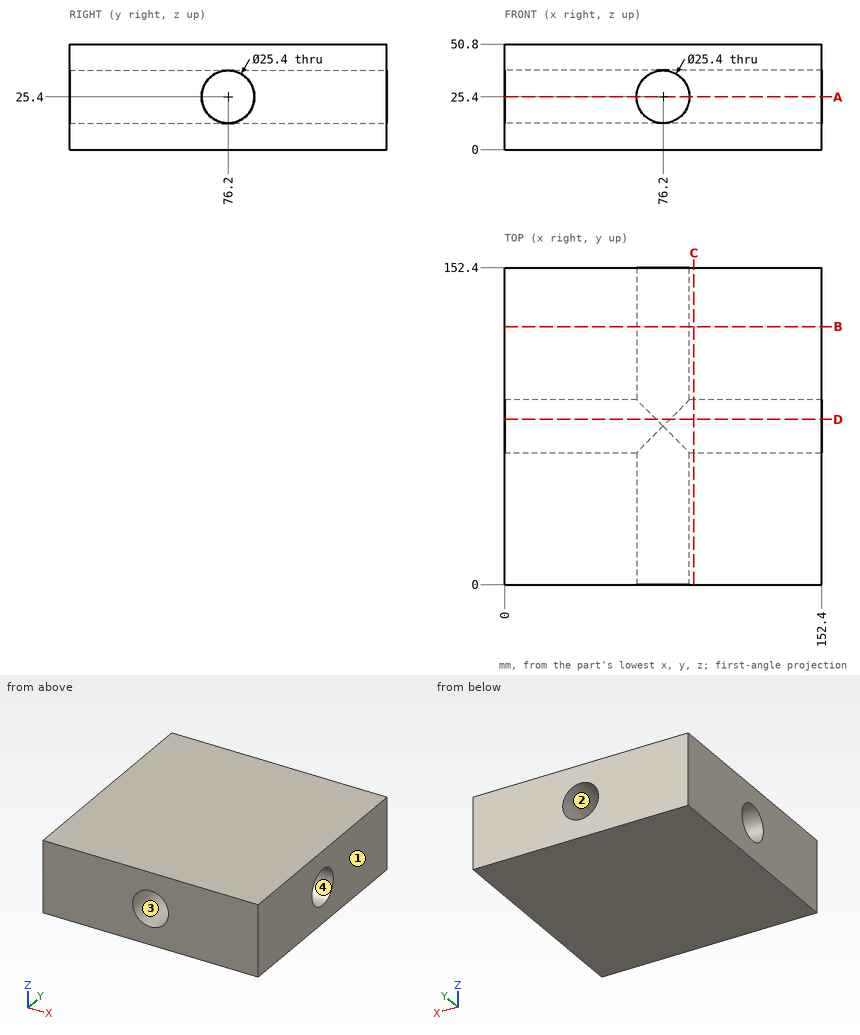
The figure shows three views and two pictorial views of one solid part (mm, origin at its lowest corner). Answer the questions. Round coordinates to 2 decimals unless told otherwise and drop trailing zeros. Order: outer loops, then holes, each group sorted by start corner. A loop starts at its lowest first (then second) coordinate and runs counter-clockwise, first axis right, second up. Notation, with made-up numbers: M -29,84 L 12,84 A19 cw 12,90 Z; hole C 71,79 d4. An arc over 180 degrees is marked long. Answer in a Markdown table with one row per item. Add a question column.
1) The part is cut by section B-B on y = 124. Determine the outline of the cut face in (x, z).
2) The part is cut by section D-D on y = 79.5. Determine the outline of the cut face in (x, z), plus the area to 3 significant figures.
3) Consider line 1 along Z through (x, y) = (76, 47); line 2 along Y through (x, z) = (35, 25); line 3 along X through (y, z) = (13.5, 16.5). Determine where each line is inside the solid, lowest interval first. Write a range as from..to.
4) The part is cut by section A-A on z = 25.4. Determine the outline of the cut face in (x, y).
5) Determine the mould class of the marked faces 1, 2, 3 and 4 for opening direction X: pulls with the +X half, pulls with the -X half, needs draft (parallel to the pull), parting line crosses it, or undercut.
Findings below:
| question | item | result |
|---|---|---|
| 1 | outline | M 0,0 L 152.4,0 L 152.4,50.8 L 0,50.8 Z; hole C 76.2,25.4 d25.4 |
| 2 | outline | M 0,0 L 152.4,0 L 152.4,13.14 L 79.5,13.14 A12.7 cw 72.9,13.14 L 0,13.14 Z; M 0,37.66 L 72.9,37.66 A12.7 cw 79.5,37.66 L 152.4,37.66 L 152.4,50.8 L 0,50.8 Z |
| 2 | area | 4,000 mm² |
| 3 | line 1 | z = 0..12.7, 38.1..50.8 |
| 3 | line 2 | y = 0..63.51, 88.89..152.4 |
| 3 | line 3 | x = 0..67.14, 85.26..152.4 |
| 4 | outline | M 0,0 L 63.5,0 L 63.5,63.5 L 0,63.5 Z; M 0,88.9 L 63.5,88.9 L 63.5,152.4 L 0,152.4 Z; M 88.9,0 L 152.4,0 L 152.4,63.5 L 88.9,63.5 Z; M 88.9,88.9 L 152.4,88.9 L 152.4,152.4 L 88.9,152.4 Z |
| 5 | face 1 | pulls with the +X half |
| 5 | face 2 | undercut |
| 5 | face 3 | undercut |
| 5 | face 4 | needs draft |
